```python
from build123d import *

# Parameters (mm, degrees)
SKETCH030_W     = 180
SKETCH030_H     = 140
PAD008_DEPTH    = 3
FILLET002_R     = 4
SKETCH031_R     = 6.5
SKETCH031_R_2   = 23.75
SKETCH031_R_3   = 4
POCKET006_DEPTH = 3.001


with BuildPart() as part:
    # Sketch030 (on XY_Plane010 of Origin021) → Pad008 (new body)
    with BuildSketch(Plane.XY):
        with Locations((2.306624, -28.831528)):
            Rectangle(SKETCH030_W, SKETCH030_H)
    extrude(amount=PAD008_DEPTH)

    # Fillet002
    fillet002_edges = [part.edges().sort_by_distance(p)[0] for p in [
        (-87.693376, 41.168472, 1.5),
        (92.306624, 41.168472, 1.5),
        (92.306624, -98.831528, 1.5),
        (-87.693376, -98.831528, 1.5),
    ]]
    fillet(fillet002_edges, radius=FILLET002_R)

    # Sketch031 (on Face5 of Fillet002) → Pocket006 (cut, through all)
    with BuildSketch(Plane.XY.offset(3)):
        with Locations((-68, 20)):
            Circle(SKETCH031_R)
        with Locations((-52, -44)):
            Circle(SKETCH031_R_2)
        with Locations((52, -44)):
            Circle(SKETCH031_R_3)
        with Locations((0, -80)):
            Circle(SKETCH031_R)
        with Locations((68, 20)):
            Circle(SKETCH031_R)
        with BuildLine():
            Line((-28.75, -4), (28.75, -4))
            ThreePointArc((28.75, -4), (29.457107, -3.707107), (29.75, -3))
            Line((29.75, -3), (29.75, 27.3))
            ThreePointArc((29.75, 27.3), (29.457107, 28.007107), (28.75, 28.3))
            Line((28.75, 28.3), (-28.75, 28.3))
            ThreePointArc((-28.75, 28.3), (-29.457107, 28.007107), (-29.75, 27.3))
            Line((-29.75, 27.3), (-29.75, -3))
            ThreePointArc((-29.75, -3), (-29.457107, -3.707107), (-28.75, -4))
        make_face()
    extrude(amount=-POCKET006_DEPTH, mode=Mode.SUBTRACT)


solid = part.part
```
Can you work these out from the model? Positions are in its coordinate system, mm. Coordinates: 2 decimals unless noted, no trailing zeros. Write each loop counter-clockwise with the first axis right and the second up, starting at its lowest first coordinate (ties: lowest second). Pieces come first, ordered by that corner, then holes. Notation, with made-up numbers: M 52,62.25 L 88,62.25 A15 ccw 88,83.25 Z; hole C -32,-32 d6. An arc over 180 degrees is marked long. Write item = value, one per line. Start each with the question number.
Q1. If we section it at C-C, the plane y = -80: Write out the boundary of the cut face in (x, z), then the cut area to 3 significant figures.
Q2. If we section it at D-D, the plane z = 2: Write out the boundary of the cut face in (x, y), then the cut area to 3 significant figures.
Q3. If I drill on L1, parallel to Y at x = 52, z = 2.6; L2, parallel to Y at x = 0, z = 1.8; L3, parallel to Y at x = -52, z = 0.8, over which ranges is the centre line in solid material (lowest first)? Write a range as [from, to].
Q4. If we section it at B-B, the plane y = -44: Write out the boundary of the cut face in (x, z), then the cut area to 4 significant figures.
Q5. If we section it at A-A, the plane x = 68: Write out the boundary of the cut face in (y, z).
Q6. Thinking about a two-plate mould opening in Y: for faces 1 (the face through (51.479, -40.034, 1.521)), 2 (the face through (91.166, 39.966, 1.521)), 3 (the face through (74.2, 21.95, 1.52)), 4 (the face through (1, -28, 0)), which applies, released by +Y, released by -Y, zero draft, split by the parting line, or undercut?
Check sheet entries:
q1.outline = M -87.69,0 L -6.5,0 L -6.5,3 L -87.69,3 Z; M 6.5,0 L 92.31,0 L 92.31,3 L 6.5,3 Z
q1.area = 501 mm²
q2.outline = M -87.69,-94.83 A4 ccw -83.69,-98.83 L 88.31,-98.83 A4 ccw 92.31,-94.83 L 92.31,37.17 A4 ccw 88.31,41.17 L -83.69,41.17 A4 ccw -87.69,37.17 Z; hole C -52,-44 d47.5; hole C -68,20 d13; hole M -29.75,-3 A1 ccw -28.75,-4 L 28.75,-4 A1 ccw 29.75,-3 L 29.75,27.3 A1 ccw 28.75,28.3 L -28.75,28.3 A1 ccw -29.75,27.3 Z; hole C 0,-80 d13; hole C 52,-44 d8; hole C 68,20 d13
q2.area = 21,000 mm²
q3.L1 = [-98.83, -48], [-40, 41.17]
q3.L2 = [-98.83, -86.5], [-73.5, -4], [28.3, 41.17]
q3.L3 = [-98.83, -67.75], [-20.25, 41.17]
q4.outline = M -87.69,0 L -75.75,0 L -75.75,3 L -87.69,3 Z; M -28.25,0 L 48,0 L 48,3 L -28.25,3 Z; M 56,0 L 92.31,0 L 92.31,3 L 56,3 Z
q4.area = 373.5 mm²
q5.outline = M -98.83,0 L 13.5,0 L 13.5,3 L -98.83,3 Z; M 26.5,0 L 41.17,0 L 41.17,3 L 26.5,3 Z
q6.face_1 = undercut
q6.face_2 = released by +Y
q6.face_3 = undercut
q6.face_4 = zero draft
